Autodesk Inventor part; units mm, degrees
ref_plane "YZ Plane" through (0, 0, 0) normal (1, 0, 0) x (0, 1, 0)
ref_plane "XZ Plane" through (0, 0, 0) normal (0, 1, 0) x (-1, 0, 0)
ref_plane "XY Plane" through (0, 0, 0) normal (0, 0, 1) x (1, 0, 0)
sketch "Sketch1" plane through (0, 0, 0) normal (0, 1, 0) x (-1, 0, 0)
  line L0 (0, 0) -> (45, 0)
  line L1 (45, 0) -> (45, -20)
  line L2 (45, -20) -> (0, -20)
  line L3 (0, -20) -> (0, 0)
  dimension "d0" = 45
  dimension "d1" = 20
extrude "Extrusion1" add sketch "Sketch1" along normal blind 4
sketch "Sketch2" plane through (0, 4, 0) normal (0, 1, 0) x (1, 0, 0)
  line L0 (0, 0) -> (0, 20)
  line L1 (-45, 20) -> (-45, 0)
  line L2 (-45, 10) -> (-35.5, 10)
  line L3 (0, 10) -> (-9.5, 10)
  circle A0 centre (-9.5, 10) radius 8
  circle A1 centre (-35.5, 10) radius 8
  line L4 (-35.5, 10) -> (-9.5, 10)
  dimension "d4" = 9.5
  dimension "d5" = 9.5
  dimension "d6" = 16
  dimension "d7" = 16
  dimension "d8" = 26
extrude "Extrusion2" add sketch "Sketch2" along normal blind 13.8
properties part number "HC-SR04"
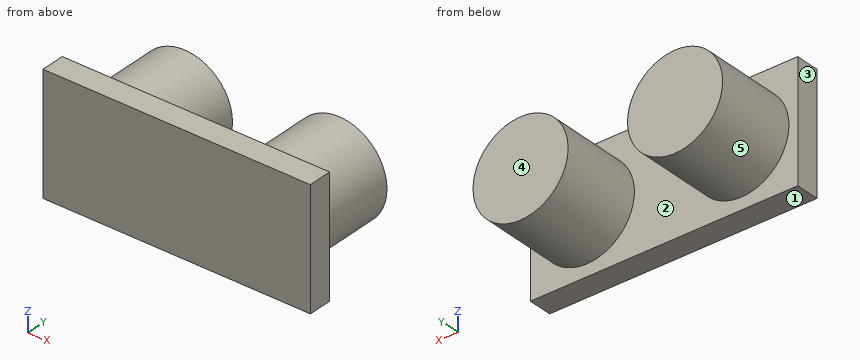
For this review, take the finished solid that the model builds, in its own axes (mm). Face numbers are marked on the shaded views. A direction names the side the tool comes from. Round coordinates to 2 decimals unless told otherwise and drop trailing zeros. Order: outer loops, then holes, each group sorted by start corner. A loop starts at its lowest first (then second) coordinate and runs counter-clockwise, first axis right, second up. Notation, with made-up numbers: M -22,85.5 L -5,85.5 A22 cw -5,102.5 Z; hole C -21,53 d10. An arc over 180 degrees is marked long. Use a Markdown table: item, result. Add a question column.
Item 1: Add section B-B, the plane z = -10. Give the boundary of the cut face in (x, y).
Item 2: Add section D-D, the plane z = -16. Give the boundary of the cut face in (x, y).
Item 3: Add section C-C, the plane x = -10.5. Give the boundary of the cut face in (y, z), then the cut area to 3 significant figures.
Item 4: Tool access review of the marked faces 4 and 5: name each direction out of +Z, -Z, +X, -X, +Y, -Y from which nothing blocks a thin tool from reaching the whole face with its end or side.
Item 5: To check wall thickness, follow line 1 along Y through (x, z) = (-26, -5.75); line 2 along X through (y, z) = (16.75, -5.5); line 3 along X through (y, z) = (15.25, -16.75). State the ranges of each line that lie inside material, in increasing order.
Item 6: Mouldability with a two-part tool opening along X and no side actions: class the marked faces 1, 2 and 3 as released by +X, released by -X, zero draft, split by the parting line, or undercut.
Item 7: Insertion check: pin 1 (10 mm diameter, centred on y = 2, z = -3.5, fed in from +X). The pin has a flat end and moves straight along its axis. Give the tip position at first contact, or say it passes through.
Item 8: Add section A-A, the plane x = -35.5. Give the boundary of the cut face in (y, z).
Geometry results:
| question | item | result |
|---|---|---|
| 1 | outline | M -45,0 L 0,0 L 0,4 L -1.5,4 L -1.5,17.8 L -17.5,17.8 L -17.5,4 L -27.5,4 L -27.5,17.8 L -43.5,17.8 L -43.5,4 L -45,4 Z |
| 2 | outline | M -45,0 L 0,0 L 0,4 L -4.21,4 L -4.21,17.8 L -14.79,17.8 L -14.79,4 L -30.21,4 L -30.21,17.8 L -40.79,17.8 L -40.79,4 L -45,4 Z |
| 3 | outline | M 0,-20 L 4,-20 L 4,-17.94 L 17.8,-17.94 L 17.8,-2.06 L 4,-2.06 L 4,0 L 0,0 Z |
| 3 | area | 299 mm² |
| 4 | face 4 | +Z, -Z, +X, -X, +Y |
| 4 | face 5 | +Y |
| 5 | line 1 | y = 0 to 4 |
| 5 | line 2 | x = -42.11 to -28.89, -16.11 to -2.89 |
| 5 | line 3 | x = -39.79 to -31.21, -13.79 to -5.21 |
| 6 | face 1 | zero draft |
| 6 | face 2 | undercut |
| 6 | face 3 | released by -X |
| 7 | pin 1 | stops at x = 0 |
| 8 | outline | M 0,-20 L 4,-20 L 4,-18 L 17.8,-18 L 17.8,-2 L 4,-2 L 4,0 L 0,0 Z |
